Model file for the job. Use its own axes, mm. A direction names the side the tool comes from. Round coordinates to 2 decimals unless told otherwise and drop trailing zeros. Loops run counter-clockwise (first coordinate to the right, second up) from the corner with the lowest first, then second, coordinate; pieces in that order, holes last. Notation, with made-up numbers: (5, 52) -> (23, 52) arc R26 ccw to (23, 90) -> close; hole circle Ø11 at (34.25, 69). An arc over 180 degrees is marked (long way). Use a Markdown table: item, result.
from build123d import *

# Parameters (mm, degrees)
F0_W      = 117
F0_H      = 60
F1_DEPTH  = 60
F2_W      = 42
F2_H      = 10
F3_DEPTH  = 117
F4_W      = 26
F4_H      = 16
F5_DEPTH  = 117
F7_DEPTH  = 22
F9_DEPTH  = 22
F11_DEPTH = 22
F13_DEPTH = 60
F15_DEPTH = 60


with BuildPart() as f1:
    # F0 (on Front) → F1 (new body)
    with BuildSketch(Plane.XZ):
        with Locations((-58.5, 30)):
            Rectangle(F0_W, F0_H)
    extrude(amount=F1_DEPTH)

    # F2 (on face) → F3 (cut)
    with BuildSketch(Plane.YZ):
        with Locations((-30, 5)):
            Rectangle(F2_W, F2_H)
    extrude(amount=-F3_DEPTH, mode=Mode.SUBTRACT)

    # F4 (on face) → F5 (cut)
    with BuildSketch(Plane.YZ):
        with Locations((-30, 18)):
            Rectangle(F4_W, F4_H)
    extrude(amount=-F5_DEPTH, mode=Mode.SUBTRACT)

    # F6 (on face) → F7 (cut)
    with BuildSketch(Plane.YZ):
        with BuildLine():
            ThreePointArc((-38, 41), (-30, 33), (-22, 41))
            ThreePointArc((-22, 41), (-30, 49), (-38, 41))
        make_face()
    extrude(amount=-F7_DEPTH, mode=Mode.SUBTRACT)

    # F8 (on face) → F9 (cut)
    with BuildSketch(Plane.YZ):
        Polygon((-44, 60), (-60, 60), (-60, 44), align=None)
    extrude(amount=-F9_DEPTH, mode=Mode.SUBTRACT)

    # F10 (on face) → F11 (cut)
    with BuildSketch(Plane.YZ):
        Polygon((0, 44), (0, 60), (-16, 60), align=None)
    extrude(amount=-F11_DEPTH, mode=Mode.SUBTRACT)

    # F12 (on face) → F13 (cut)
    with BuildSketch(Plane.XZ.offset(60)):
        Polygon((-22, 60), (-88, 60), (-88, 26), (-22, 26), (-22, 44), align=None)
    extrude(amount=-F13_DEPTH, mode=Mode.SUBTRACT)

    # F14 (on face) → F15 (cut)
    with BuildSketch(Plane.XZ.offset(60)):
        Polygon((-101, 60), (-117, 60), (-117, 44), align=None)
    extrude(amount=-F15_DEPTH, mode=Mode.SUBTRACT)


solid = f1.part
Q1. Pull direction X, two halves, no side cores. Call faces 4 (the face through (0, -30, 30)), 5 (the face through (-11, -8, 52)), 6 (the face through (-109, -30, 52)), 7 (the face through (-55, -52, 26)): released by +X, released by -X, zero draft, split by the parting line, or undercut.
Results list:
| item | result |
|---|---|
| face 4 | released by +X |
| face 5 | zero draft |
| face 6 | released by -X |
| face 7 | undercut |
Q2. Band-saw the part on A-A, the plane y = -30. Give the cut face in (x, z), plus the area to 3 significant figures.
Results list:
| item | result |
|---|---|
| outline | (-117, 26) -> (-88, 26) -> (-88, 60) -> (-101, 60) -> (-117, 44) -> close; (-22, 26) -> (0, 26) -> (0, 33) -> (-22, 33) -> close; (-22, 49) -> (0, 49) -> (0, 60) -> (-22, 60) -> close |
| area | 1,250 mm² |
Q3. Tool access for faces 1 (the face through (-58, -9, 5)), 2 (the face through (-11, -52, 52)), 3 (the face through (-22, -24, 47)): list every direction of +Z, -Z, +X, -X, +Y, -Y with a clear straight run to the whole face (end or side of a thin tool).
Results list:
| item | result |
|---|---|
| face 1 | -Z, +X, -X |
| face 2 | +Z, +X, -Y |
| face 3 | +Z, +Y, -Y |
Q4. Band-saw the part on D-D, the plane y = -19. Give the cut face in (x, z).
Results list:
| item | result |
|---|---|
| outline | (-117, 26) -> (-88, 26) -> (-88, 60) -> (-101, 60) -> (-117, 44) -> close; (-22, 26) -> (0, 26) -> (0, 60) -> (-22, 60) -> close |
Q5. Band-saw the part on B-B, the plane x = -44.5. Give the cut face in (y, z), plus the area to 3 significant figures.
Results list:
| item | result |
|---|---|
| outline | (-60, 0) -> (-51, 0) -> (-51, 10) -> (-43, 10) -> (-43, 26) -> (-60, 26) -> close; (-17, 10) -> (-9, 10) -> (-9, 0) -> (0, 0) -> (0, 26) -> (-17, 26) -> close |
| area | 724 mm² |
Q6. Band-saw the part on C-C, the plane z = 17. Give the cut face in (x, y), plus the area to 3 significant figures.
Results list:
| item | result |
|---|---|
| outline | (-117, -60) -> (0, -60) -> (0, -43) -> (-117, -43) -> close; (-117, -17) -> (0, -17) -> (0, 0) -> (-117, 0) -> close |
| area | 3,980 mm² |
Q7. Flat gauge pins, fed straight in: pin 1 (2.5 mm diameter, centred on x = -87, y = -49, fed in from -Z); pin 2 (18.5 mm diameter, centred on x = -49, y = -55.5, fed in from +Z); pin 3 (6.5 mm diameter, centred on x = -15.5, y = -26.5, fed in from -Z). Where does each tip first touch, or does it go through?
Results list:
| item | result |
|---|---|
| pin 1 | stops at z = 10 |
| pin 2 | stops at z = 26 |
| pin 3 | stops at z = 26 |
Q8. Drill centre lines: L1, parallel to Z at x = -16, y = -30; L2, parallel to Y at x = -69.5, z = 17.5; L3, parallel to X at y = -49, z = 43.5. Where is each one in solid material? Low to high. Write a range as from..to.
Results list:
| item | result |
|---|---|
| L1 | z = 26..33, 49..60 |
| L2 | y = -60..-43, -17..0 |
| L3 | x = -117..-88, -22..0 |
